```python
from build123d import *

# Parameters (mm, degrees)
SKETCH1_R           = 4.826
BOSS_EXTRUDE1_DEPTH = 180.34
SKETCH2_R           = 3.4925
BOSS_EXTRUDE2_DEPTH = 1.27
SKETCH3_R           = 3.49123
CUT_EXTRUDE2_DEPTH  = 203.2


with BuildPart() as part:
    # Sketch1 → Boss-Extrude1 (new body)
    with BuildSketch(Plane(origin=(0, 0, 0), x_dir=(1, 0, 0), z_dir=(0, 1, 0))):
        with Locations(Location((0, 0, 0), (0, 0, 270))):
            Circle(SKETCH1_R)
    extrude(amount=BOSS_EXTRUDE1_DEPTH)

    # Sketch2 → Boss-Extrude2 (add)
    with BuildSketch(Plane(origin=(0, 180.34, 0), x_dir=(1, 0, 0), z_dir=(0, 1, 0))):
        with Locations(Location((0, 0, 0), (0, 0, 270))):
            Circle(SKETCH2_R)
    extrude(amount=BOSS_EXTRUDE2_DEPTH)

    # loft from a face of the part (loft3)
    loft([part.faces().sort_by_distance((0, 181.61, 0))[0], Face(Wire([part.edges().sort_by_distance((3.518002596, 180.34, -3.303624333))[0]]))])

    # Sketch3 → Cut-Extrude2 (cut)
    with BuildSketch(Plane(origin=(0, 181.61, 0), x_dir=(1, 0, 0), z_dir=(0, 1, 0))):
        with Locations(Location((0, 0, 0), (0, 0, 270))):
            Circle(SKETCH3_R)
    extrude(amount=-CUT_EXTRUDE2_DEPTH, mode=Mode.SUBTRACT)


solid = part.part
```
Source: CAD feature listing. Evaluate the final solid. Frame: model axes, mm. Coordinates: 2 decimals unless noted, no trailing zeros. Loops run counter-clockwise (first coordinate to the right, second up) from the corner with the lowest first, then second, coordinate; pieces in that order, holes last. Notation, with made-up numbers: M -15.5,-20.75 L 14.5,-20.75 A25 ccw 14.5,-3.75 Z; hole C 10.5,63 d3. An arc over 180 degrees is marked long. Use CSV: the item, a comma, the result in double quotes.
(1) Draft query along X for faces 1 (the face through (3, 0, -3)), 2 (the face through (-2.937, 88.908, -3.83)), 3 (the face through (-3.4, 92.1, -0.8)). Return one class per face: pulls with the +X half, pulls with the -X half, needs draft (parallel to the pull), parting line crosses it, or undercut.
Answers follow:
face 1,"needs draft"
face 2,"parting line crosses it"
face 3,"undercut"
(2) Contact query for flat-ended pins moving along their axis: pin 1 (4 mm diameter, centred on x = 2, z = -3, fed in from -Y); pin 2 (3 mm diameter, centred on x = 3.5, y = 114, fed in from -Z); pin 3 (4 mm diameter, centred on y = 19.5, z = 3, fed in from -X); pin 4 (1.5 mm diameter, centred on y = 130.5, z = -3.5, fed in from +X). Output: stop coordinate, or through.
Answers follow:
pin 1,"y = 0"
pin 2,"z = -4.39"
pin 3,"x = -4.72"
pin 4,"x = 3.97"
(3) Line query: line 1 (X direction, y = 123.5, z = 0); line 2 (Z direction, x = 2, y = 103); line 3 (Z direction, x = -1.5, y = 50). Output: solid intervals per line, ascending. Write a range as [from, to].
Answers follow:
line 1,"[-4.83, -3.49], [3.49, 4.83]"
line 2,"[-4.39, -2.86], [2.86, 4.39]"
line 3,"[-4.59, -3.15], [3.15, 4.59]"
(4) Cut plane B-B on y = 142.5. Return loops of the section in (x, z).
Answers follow:
outline,"C 0,0 d9.65; hole C 0,0 d6.98"
